Design review of the part shown in the three views and the two pictorial views. Dimensions are in mm from the part's minimum x, y and z. Coordinates: 2 decimals unless noted, no trailing zeros. Loops run counter-clockwise (first coordinate to the right, second up) from the corner with the lowest first, then second, coordinate; pieces in that order, holes last. Notation, with made-up numbers: (70.5, -3.5) - (104.5, -3.5) arc R16 ccw to (104.5, 19.5) - close; hole circle Ø9 at (64.5, 86.5). An arc over 180 degrees is marked (long way). One line per item, written item: value. Start each with the question number.
1. To check wall thickness, follow line 1 (Y direction, x = 127, z = 5.75) (1 decimal); line 2 (X direction, y = 88.5, z = 3); line 3 (X direction, y = 114, z = 5.75). State the ranges of each line that lie inside material, in increasing order. Write a range as from..to.
2. Take a section at B-B, the plane y = 35. State the section outline as (x, z) points, and give its area (3 significant figures).
3. Insertion check: pin 1 (1.9 mm diameter, centred on y = 2.5, z = 2.5, fed in from -X); pin 2 (1.9 mm diameter, centred on y = 44.5, z = 3.5, fed in from +X). Each pin has a flat end and moves straight along its axis. Give the tip position at first contact, or say it passes through.
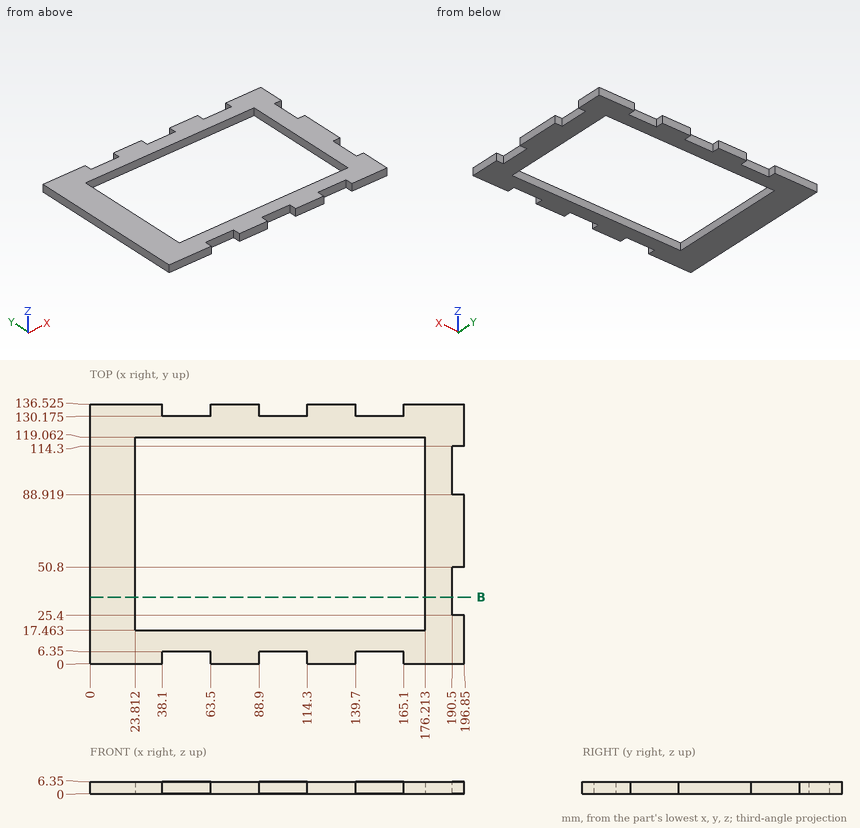
Solutions:
1. line 1: 0..17.5, 119.1..136.5
1. line 2: 0..23.81, 176.21..196.85
1. line 3: 0..23.81, 176.21..190.5
2. outline: (0, 0) - (23.81, 0) - (23.81, 6.35) - (0, 6.35) - close; (176.21, 0) - (190.5, 0) - (190.5, 6.35) - (176.21, 6.35) - close
2. area: 242 mm2
3. pin 1: x = 0
3. pin 2: x = 190.5
